For this review, take the finished solid that the model builds, in its own axes (mm). Coordinates: 2 decimals unless noted, no trailing zeros. Order: outer loops, then holes, each group sorted by start corner. A loop starts at its lowest first (then second) coordinate and runs counter-clockwise, first axis right, second up. Notation, with made-up numbers: (86, 26) -> (91, 26) arc R19 cw to (91, 40) -> close; hole circle Ø4 at (9.25, -5). An arc over 180 degrees is marked (long way). Write item = value, one per line. Start each with the question number.
1) Consider section D-D on x = 5. Give the boundary of the cut face in (y, z).
2) Wall thickness on probe 1 along Z at (x, y) = (5, 7); probe 2 along Z at (x, y) = (5, 12); probe 3 along X at (y, z) = (5, -57): over which ranges is each line inside the solid? List them lowest first. Write a range as [from, to].
3) Consider section A-A on y = 8. Give the boundary of the cut face in (x, z).
4) Consider section C-C on y = 24. Give the boundary of the cut face in (x, z).
5) Insertion check: pin 1 Ø2.5 at (x, z) = (9, 57) entering from +Y; pin 2 Ø6 at (x, y) = (2.5, 25) entering from -Z; pin 3 Ø5 at (x, z) = (6, 24.5) entering from +Y. Each pin has a flat end and moves straight along its axis. Give the tip position at first contact, or say it passes through.
6) Consider section B-B on z = 57. Give the boundary of the cut face in (x, y).
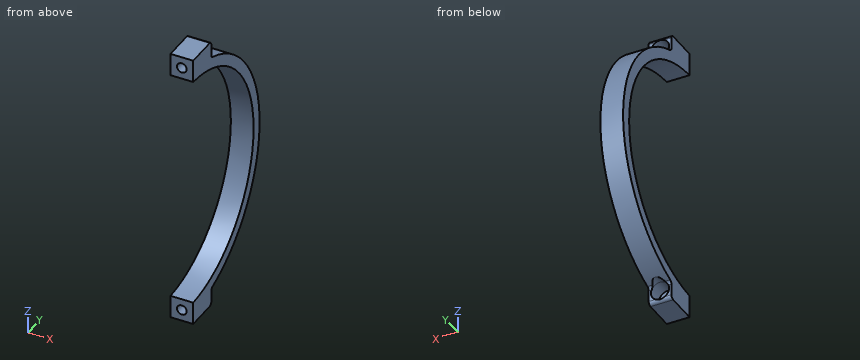
from build123d import *

# Parameters (mm, degrees)
BOSS_EXTRUDE1_DEPTH                        = 10
CBORE_FOR_M4_CHEESE_HEAD_SCREW1_AT_2_COUNT = 2
CBORE_FOR_M4_CHEESE_HEAD_SCREW1_AT_2_PITCH = 114
SKETCH6_R                                  = 4
CUT_EXTRUDE1_DEPTH                         = 8


with BuildPart() as part:
    # Sketch1 → Boss-Extrude1 (new body)
    with BuildSketch(Plane(origin=(0, 0, 0), x_dir=(0, 0, -1), z_dir=(1, 0, 0))):
        with BuildLine():
            Line((-62, 2), (-51.961524227, 2))
            ThreePointArc((-51.961524227, 2), (0, 52), (51.961524227, 2))
            Line((51.961524227, 2), (62, 2))
            Line((62, 2), (62, 15.5))
            ThreePointArc((62, 15.5), (61.560660172, 16.560660172), (60.5, 17))
            Line((60.5, 17), (55.497747702, 17))
            ThreePointArc((55.497747702, 17), (54.620689683, 17.283131383), (54.07472853, 18.025641026))
            ThreePointArc((54.07472853, 18.025641026), (0, 57), (-54.07472853, 18.025641026))
            ThreePointArc((-54.07472853, 18.025641026), (-54.620689683, 17.283131383), (-55.497747702, 17))
            Line((-55.497747702, 17), (-60.5, 17))
            ThreePointArc((-60.5, 17), (-61.560660172, 16.560660172), (-62, 15.5))
            Line((-62, 15.5), (-62, 2))
        make_face()
    extrude(amount=BOSS_EXTRUDE1_DEPTH)

    # Sketch4 → CBORE for M4 Cheese Head Screw1 (revolve, cut)
    with BuildSketch(Plane(origin=(5, 17, -57), x_dir=(0, 0, 1), z_dir=(1, 0, 0))):
        Polygon((0, 0), (0, 21.291850331), (2.15, 20), (2.15, 6.6), (4, 6.6), (4, 0), align=None)
    cbore_for_m4_cheese_head_screw1 = revolve(axis=Axis((5, 23.35, -57), (0, -1, 0)), mode=Mode.SUBTRACT)

    # CBORE for M4 Cheese Head Screw1 at 2: CBORE for M4 Cheese Head Screw1 ×2
    with Locations(*[(0, 0, i * CBORE_FOR_M4_CHEESE_HEAD_SCREW1_AT_2_PITCH) for i in range(1, CBORE_FOR_M4_CHEESE_HEAD_SCREW1_AT_2_COUNT)]):
        add(cbore_for_m4_cheese_head_screw1, mode=Mode.SUBTRACT)

    # Sketch6 → Cut-Extrude1 (cut)
    with BuildSketch(Plane(origin=(0, 17, 0), x_dir=(1, 0, 0), z_dir=(0, 1, 0))):
        with Locations((5, 57)):
            Circle(SKETCH6_R)
        with Locations((5, -57)):
            Circle(SKETCH6_R)
    extrude(amount=CUT_EXTRUDE1_DEPTH, mode=Mode.SUBTRACT)


solid = part.part
Answer sheet:
q1.outline = (2, -62) -> (15.5, -62) arc R1.5 ccw to (16.91, -61) -> (10.4, -61) -> (10.4, -59.15) -> (2, -59.15) -> close; (2, -54.85) -> (10.4, -54.85) -> (10.4, -53) -> (20.98, -53) arc R57 ccw to (20.98, 53) -> (10.4, 53) -> (10.4, 54.85) -> (2, 54.85) -> (2, 51.96) arc R52 cw to (2, -51.96) -> close; (2, 59.15) -> (10.4, 59.15) -> (10.4, 61) -> (16.91, 61) arc R1.5 ccw to (15.5, 62) -> (2, 62) -> close
q2.probe_1 = [-62, -59.15], [-54.85, -51.53], [51.53, 54.85], [59.15, 62]
q2.probe_2 = [-62, -61], [-53, -50.6], [50.6, 53], [61, 62]
q2.probe_3 = [0, 2.85], [7.15, 10]
q3.outline = (0, -62) -> (10, -62) -> (10, -51.38) -> (0, -51.38) -> close; (0, 51.38) -> (10, 51.38) -> (10, 62) -> (0, 62) -> close; hole circle Ø4.3 at (5, -57); hole circle Ø4.3 at (5, 57)
q4.outline = (0, -51.7) -> (10, -51.7) -> (10, -46.13) -> (0, -46.13) -> close; (0, 46.13) -> (10, 46.13) -> (10, 51.7) -> (0, 51.7) -> close
q5.pin_1 = 17
q5.pin_2 = -52.58
q5.pin_3 = 52.58
q6.outline = (0, 2) -> (2.85, 2) -> (2.85, 10.4) -> (1, 10.4) -> (1, 17) -> (0, 17) -> close; (7.15, 2) -> (10, 2) -> (10, 17) -> (9, 17) -> (9, 10.4) -> (7.15, 10.4) -> close
